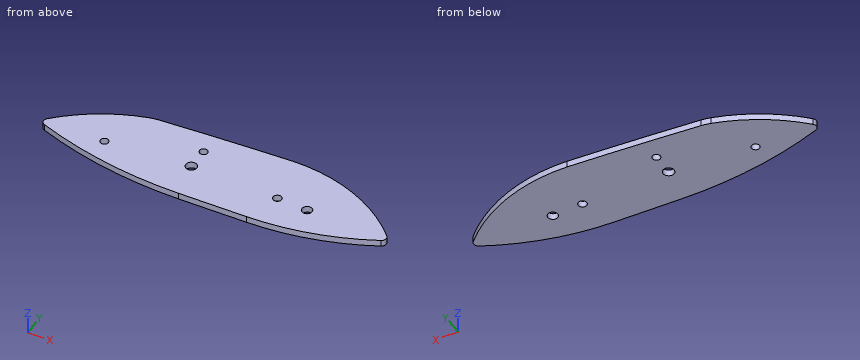
```python
from build123d import *

# Parameters (mm, degrees)
F0_R     = 4.025
F0_R_2   = 5.5
F0_R_3   = 4.25
F0_R_4   = 5
F0_R_5   = 4
F1_DEPTH = 6.35


# Not quite as in the source:
# - a length typed as a fraction of an inch, garbled in the dataset ("3 / 203.2 mm" for 3/8 in), is restored


with BuildPart() as f1:
    # F0 (on Top) → F1 (new body)
    with BuildSketch(Plane.XY):
        with BuildLine():
            ThreePointArc((7.0672459204, -2.7674484319), (79.7907725168, -23.1351403858), (155, -30))
            Line((155, -30), (222, -30))
            ThreePointArc((222, -30), (283.0205715955, -23.1551675229), (341.0080980578, -2.9608944665))
            ThreePointArc((341.0080980578, -2.9608944665), (343.7637603339, 0.6365005197), (342.4812933157, 4.982786706))
            ThreePointArc((342.4812933157, 4.982786706), (287.5845162749, 43.1113755357), (222, 56))
            ThreePointArc((222, 56), (157.0912257731, 53.5938902672), (92.2239851956, 50.2503239761))
            ThreePointArc((92.2239851956, 50.2503239761), (87.6396110054, 49.7679486163), (83.1191443173, 48.8654223701))
            ThreePointArc((83.1191443173, 48.8654223701), (41.3356630681, 32.3684999851), (5.3506191001, 5.478271944))
            ThreePointArc((5.3506191001, 5.478271944), (3.9527325419, 0.8857070849), (7.0672459204, -2.7674484319))
        make_face()
        with Locations((64, 2)):
            Circle(F0_R, mode=Mode.SUBTRACT)
        with Locations((147, 8)):
            Circle(F0_R_2, mode=Mode.SUBTRACT)
        with Locations((234, 5)):
            Circle(F0_R_3, mode=Mode.SUBTRACT)
        with Locations((264.5, 3)):
            Circle(F0_R_4, mode=Mode.SUBTRACT)
        with Locations((147, 30.5)):
            Circle(F0_R_5, mode=Mode.SUBTRACT)
    extrude(amount=F1_DEPTH)


solid = f1.part
```
For this review, take the finished solid that the model builds, in its own axes (mm). Round coordinates to 2 decimals unless told otherwise and drop trailing zeros. Write each loop counter-clockwise with the first axis right and the second up, starting at its lowest first coordinate (ties: lowest second). Pieces come first, ordered by that corner, then holes. Notation, with made-up numbers: (33.25, 43.25) - (39.25, 43.25) arc R30 ccw to (39.25, 65.25) - close; hole circle Ø10 at (-17, 32). An arc over 180 degrees is marked (long way). Put each result on its own line as item: value.
Q1. Insertion check: pin 1 Ø13.5 at (x, y) = (234, 5) entering from +Z; pin 2 Ø6.5 at (x, y) = (147, 8) entering from +Z; pin 3 Ø1.5 at (y, z) = (5, 2) entering from -X. Each pin has a flat end and moves straight along its axis. Give the tip position at first contact, or say it passes through.
Solved:
pin 1: stops at z = 6.35
pin 2: passes through
pin 3: stops at x = 4.43
Q2. Wall thickness on probe 1 along Y at (x, z) = (147, 4.5); probe 2 along X at (y, z) = (0, 1.75); probe 3 along X at (y, z) = (34, 2.5): over which ranges is each line inside the solid? List them lowest first.
Solved:
probe 1: y = -29.92 to 2.5, 13.5 to 26.5, 34.5 to 53.14
probe 2: x = 4.22 to 60.51, 67.49 to 260.5, 268.5 to 343.6
probe 3: x = 44.33 to 145.06, 148.94 to 305.83
Q3. We need section D-D (x = 109). Give the boundary of the cut face in (y, z).
Solved:
outline: (-27.45, 0) - (51.21, 0) - (51.21, 6.35) - (-27.45, 6.35) - close
Q4. We need section A-A (z = 4.25). Count the separate pieces of the cut face and the enclosed holes in it, and give its area (3 significant figures).
Solved:
separate pieces: 1
enclosed holes: 5
area: 22,100 mm2
Q5. We need section B-B (y = 30.5). Give the boundary of the cut face in (x, z), and give its area (3 significant figures).
Solved:
outline: (38.07, 0) - (143, 0) - (143, 6.35) - (38.07, 6.35) - close; (151, 0) - (311.58, 0) - (311.58, 6.35) - (151, 6.35) - close
area: 1,690 mm2
Q6. We need section C-C (x = 264.5). Give the boundary of the cut face in (y, z).
Solved:
outline: (-26.7, 0) - (-2, 0) - (-2, 6.35) - (-26.7, 6.35) - close; (8, 0) - (50.91, 0) - (50.91, 6.35) - (8, 6.35) - close
